```python
from build123d import *

# Parameters (mm, degrees)
SKETCH1_W           = 170
SKETCH1_H           = 170
SKETCH1_R           = 1.98
BOSS_EXTRUDE1_DEPTH = 2.54
SKETCH2_W           = 158.75
SKETCH2_H           = 27
BOSS_EXTRUDE2_DEPTH = 39
SKETCH4_W           = 13.87
SKETCH4_H           = 170
BOSS_EXTRUDE3_DEPTH = 16
SKETCH6_W           = 156.13
SKETCH6_H           = 30
BOSS_EXTRUDE4_DEPTH = 38
SKETCH5_W           = 156.13
SKETCH5_H           = 115
BOSS_EXTRUDE5_DEPTH = 57


with BuildPart() as part:
    # Sketch1 → Boss-Extrude1 (new body)
    with BuildSketch(Plane.XY):
        Rectangle(SKETCH1_W, SKETCH1_H)
        with Locations((-78.65, 74.84)):
            Circle(SKETCH1_R, mode=Mode.SUBTRACT)
        with Locations((78.83, 51.98)):
            Circle(SKETCH1_R, mode=Mode.SUBTRACT)
        with Locations((-78.65, -80.1)):
            Circle(SKETCH1_R, mode=Mode.SUBTRACT)
        with Locations((78.83, -80.1)):
            Circle(SKETCH1_R, mode=Mode.SUBTRACT)
    extrude(amount=BOSS_EXTRUDE1_DEPTH)

    # Sketch2 → Boss-Extrude2 (add)
    with BuildSketch(Plane.XY.offset(2.54)):
        with Locations((8.245, 73.5)):
            Rectangle(SKETCH2_W, SKETCH2_H)
    extrude(amount=BOSS_EXTRUDE2_DEPTH)

    # Sketch4 → Boss-Extrude3 (add)
    with BuildSketch(Plane.XY.offset(2.54)):
        with Locations((-78.065, 0)):
            Rectangle(SKETCH4_W, SKETCH4_H)
    extrude(amount=BOSS_EXTRUDE3_DEPTH)

    # Sketch6 → Boss-Extrude4 (add)
    with BuildSketch(Plane.XY.offset(2.54)):
        with Locations((6.935, -70)):
            Rectangle(SKETCH6_W, SKETCH6_H)
    extrude(amount=BOSS_EXTRUDE4_DEPTH)

    # Sketch5 → Boss-Extrude5 (add)
    with BuildSketch(Plane.XY.offset(2.54)):
        with Locations((6.935, 2.5)):
            Rectangle(SKETCH5_W, SKETCH5_H)
    extrude(amount=BOSS_EXTRUDE5_DEPTH)


solid = part.part
```
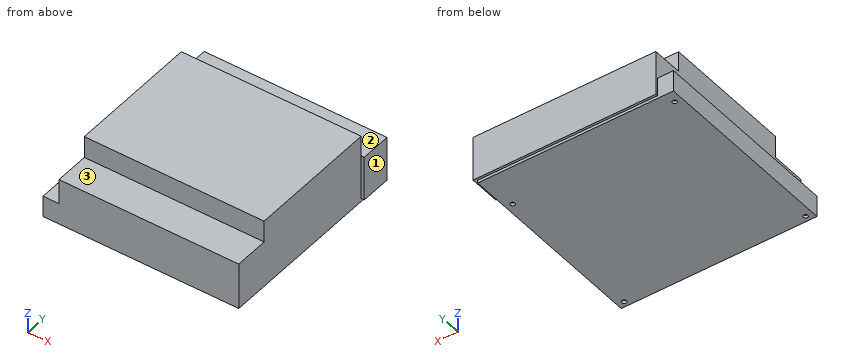
Here's how the part is built. I have some questions about the finished solid (model axes, mm). Face numbers are marked on the shaded views. A direction names the side the tool comes from. Coordinates: 2 decimals unless noted, no trailing zeros. Order: outer loops, then holes, each group sorted by start corner. A loop starts at its lowest first (then second) coordinate and runs counter-clockwise, first axis right, second up.
1) I need wall thicknesses on line 1 (Y direction, x = 78.83, z = 0.6); line 2 (X direction, y = -80, z = 1); line 3 (Y direction, x = -78.65, z = 0.8). Which ranges of each line are inside material? Lowest first, please.
2) Which directions (+Z, -Z, +X, -X, +Y, -Y) give clear straight access to the entire face, cutting with the end or side of a thin tool? Please do the marked faces 1, 2 and 3.
3) Imagine slicing it at B-B on x = 44. List the corners of the cut face in (y, z) for me.
4) Imagine slicing it at C-C on z = 38.5. List the corners of the cut face in (x, y) for me.
5) Imagine slicing it at A-A on y = -5. List the corners of the cut face in (x, z) for me, and give its area (3 significant figures).
6) Will these pins go through, and if not, where does the flat tip stop? pin 1 (4 mm diameter, centred on y = -54.5, z = 11.5, fed in from +X); pin 2 (21.5 mm diameter, centred on x = 6.5, y = 78, fed in from +Z); pin 3 (2 mm diameter, centred on x = -79, y = 75, fed in from -Z).
Response values:
1. line 1: y = -85 to -82.08, -78.12 to 50, 53.96 to 85
1. line 2: x = -85 to -80.63, -76.67 to 76.85, 80.81 to 85
1. line 3: y = -85 to -82.08, -78.12 to 72.86, 76.82 to 85
2. face 1: +Z, -Z, +X, +Y, -Y
2. face 2: +Z, +X, -X, +Y
2. face 3: +Z, +X, -X, -Y
3. outline: (-85, 0) - (85, 0) - (85, 2.54) - (87, 2.54) - (87, 41.54) - (60, 41.54) - (60, 59.54) - (-55, 59.54) - (-55, 40.54) - (-85, 40.54) - close
4. outline: (-71.13, -85) - (85, -85) - (85, 60) - (87.62, 60) - (87.62, 87) - (-71.13, 87) - close
5. outline: (-85, 0) - (85, 0) - (85, 59.54) - (-71.13, 59.54) - (-71.13, 18.54) - (-85, 18.54) - close
5. area: 9,550 mm2
6. pin 1: stops at x = 85
6. pin 2: stops at z = 41.54
6. pin 3: stops at z = 2.54
